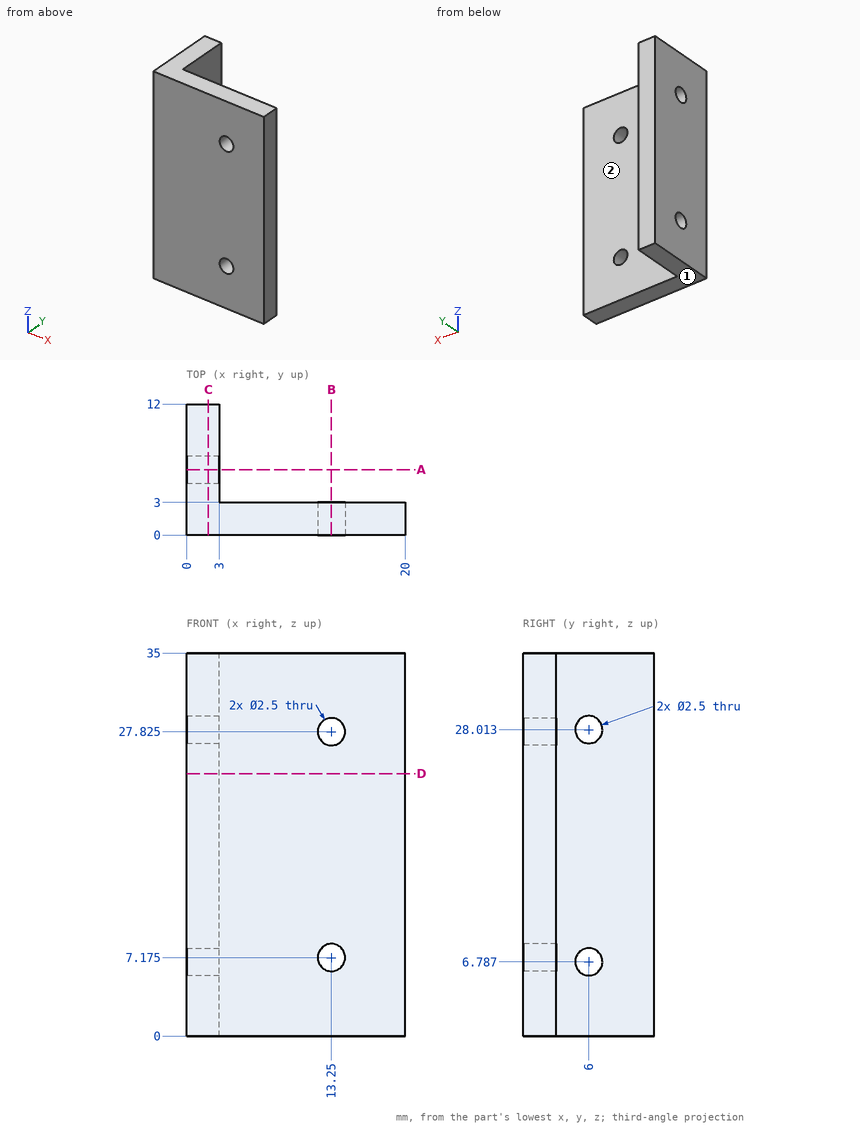
The drawing under review shows one solid part. Ordinate dimensions are in mm from its lowest x, y, z. A direction names the side the tool comes from. Round coordinates to 2 decimals unless told otherwise and drop trailing zeros. Order: outer loops, then holes, each group sorted by start corner. A loop starts at its lowest first (then second) coordinate and runs counter-clockwise, first axis right, second up. Notation, with made-up numbers: (-20, 31.25) -> (-3, 31.25) arc R10 ccw to (-3, 37.25) -> close; hole circle Ø10 at (76, -29.75). An arc over 180 degrees is marked (long way). Use a Markdown table: item, result.
Q1. We need section B-B on x = 13.25. Write out the cut boundary in (y, z) (1 decimal).
Values:
| item | result |
|---|---|
| outline | (0, 0) -> (3, 0) -> (3, 5.9) -> (0, 5.9) -> close; (0, 8.4) -> (3, 8.4) -> (3, 26.6) -> (0, 26.6) -> close; (0, 29.1) -> (3, 29.1) -> (3, 35) -> (0, 35) -> close |
Q2. Tool access review of the marked faces 1 and 2: name each direction out of +Z, -Z, +X, -X, +Y, -Y from which nothing blocks a thin tool from reaching the whole face with its end or side.
Values:
| item | result |
|---|---|
| face 1 | -Z, +X, -X, +Y, -Y |
| face 2 | +Z, -Z, +X, +Y |
Q3. We need section C-C on x = 2. Write out the cut boundary in (y, z), then the cut area to 3 significant figures.
Values:
| item | result |
|---|---|
| outline | (0, 0) -> (12, 0) -> (12, 35) -> (0, 35) -> close; hole circle Ø2.5 at (6, 6.79); hole circle Ø2.5 at (6, 28.01) |
| area | 410 mm^2 |
Q4. Clearance check with flat-ended pins moving along their axes: P1, Ø2, axis at x = 14.5, z = 13, coming from the +Y side; P2, Ø4.5, axis at y = 6.5, z = 11, coming from the +X side. State where each tip first meets the part, or that it passes through.
Values:
| item | result |
|---|---|
| P1 | stops at y = 3 |
| P2 | stops at x = 3 |
Q5. We need section A-A on y = 6. Write out the cut boundary in (x, z).
Values:
| item | result |
|---|---|
| outline | (0, 0) -> (3, 0) -> (3, 5.54) -> (0, 5.54) -> close; (0, 8.04) -> (3, 8.04) -> (3, 26.76) -> (0, 26.76) -> close; (0, 29.26) -> (3, 29.26) -> (3, 35) -> (0, 35) -> close |
Q6. For line 1 (Z direction, x = 13.25, y = 1.95) (1 decimal); line 2 (Y direction, x = 9.5, z = 13.5), list the stretches that pass through material, from the lowest coordinate up.
Values:
| item | result |
|---|---|
| line 1 | z = 0 to 5.9, 8.4 to 26.6, 29.1 to 35 |
| line 2 | y = 0 to 3 |
Q7. We need section D-D on z = 24. Write out the cut boundary in (x, y).
Values:
| item | result |
|---|---|
| outline | (0, 0) -> (20, 0) -> (20, 3) -> (3, 3) -> (3, 12) -> (0, 12) -> close |
